Design review of the part built by this model. Coordinates are the model's own, in mm. Round coordinates to 2 decimals unless told otherwise and drop trailing zeros. Order: outer loops, then holes, each group sorted by start corner. A loop starts at its lowest first (then second) coordinate and runs counter-clockwise, first axis right, second up. Notation, with made-up numbers: M 75.25,5 L 82.25,5 A26 ccw 82.25,29 Z; hole C 5.5,58.25 d1. An arc over 180 degrees is marked long. Write item = value, one per line. Start each with the question number.
```python
from build123d import *

# Parameters (mm, degrees)
F1_DEPTH = 5
F1_TAPER = 45


with BuildPart() as f1:
    # F0 (on Top) → F1 (new body)
    with BuildSketch(Plane.XY):
        Polygon((0, 29.7006979173), (-13.9796594971, 11.482050957), (-13.9796594971, -11.482050957), (0, -29.7006979173), (13.9796594971, -11.482050957), (13.9796594971, 11.482050957), align=None)
    extrude(amount=F1_DEPTH, taper=F1_TAPER)

    # F2: F1 across plane


with BuildPart() as f1_1:
    add(f1.part)
    add(f1.part.mirror(Plane.XY))


solid = f1_1.part
```
(1) For line 1 along X through (y, z) = (0, -2.5); line 2 along Y through (x, z) = (-5.5, 0.5); line 3 along Z through (x, y) = (-12.5, -10.5), list the stretches that pass through material, from the lowest coordinate up. Write a range as [from, to].
(2) Consider section C-C, the plane y = 25.5. Write out the cut boundary in (x, z).
(3) Insertion check: pin 1 (4 mm diameter, centred on y = -16, z = 3, fed in from +X); pin 2 (2 mm diameter, centred on x = 10.5, z = 0, fed in from +Y); pin 3 (3 mm diameter, centred on x = -5, z = 3.5, fed in from +Y); pin 4 (8 mm diameter, centred on x = -5.5, y = 17.5, fed in from +Z). Each pin has a flat end and moves straight along its axis. Give the tip position at first contact, or say it passes through.
(4) Consider section B-B, the plane z = -3. Write out the cut boundary in (x, y), then the cut area to 3 significant figures.
(5) Consider section A-A, the plane y = 6. Write out the cut boundary in (x, z), then the cut area to 3 significant figures.
Completed:
q1.line_1 = [-11.48, 11.48]
q1.line_2 = [-21.71, 21.71]
q1.line_3 = [-1.48, 1.48]
q2.outline = M -3.22,0 L 0,-2.56 L 3.22,0 L 0,2.56 Z
q3.pin_1 = 9.68
q3.pin_2 = 17.32
q3.pin_3 = 20.58
q3.pin_4 = 5
q4.outline = M -10.98,-10.46 L 0,-24.77 L 10.98,-10.46 L 10.98,10.46 L 0,24.77 L -10.98,10.46 Z
q4.area = 774 mm2
q5.outline = M -13.98,0 L -8.98,-5 L 8.98,-5 L 13.98,0 L 8.98,5 L -8.98,5 Z
q5.area = 230 mm2
